Autodesk Inventor part; units mm, degrees
ref_plane "YZ Plane" through (0, 0, 0) normal (1, 0, 0) x (0, 1, 0)
ref_plane "XZ Plane" through (0, 0, 0) normal (0, 1, 0) x (-1, 0, 0)
ref_plane "XY Plane" through (0, 0, 0) normal (0, 0, 1) x (1, 0, 0)
sketch "Sketch1" plane through (0, 0, 0) normal (0, 1, 0) x (-1, 0, 0)
  line L0 (60, -75) -> (-60, -75)
  line L1 (-60, 75) -> (60, -75) construction
  line L2 (60, 75) -> (-60, -75) construction
  line L3 (-60, -75) -> (-60, -55)
  line L4 (-60, -42.5) -> (-60, -55)
  line L5 (0, 75) -> (0, 40)
  line L6 (-60, -75) -> (-60, -5)
  line L7 (-30, 40) -> (-30, 10)
  line L8 (-30, 10) -> (-60, 0)
  line L9 (30, 40) -> (30, 10)
  line L10 (30, 10) -> (60, -5)
  line L11 (-30, 40) -> (-30, 48)
  line L12 (30, 40) -> (30, 48)
  line L13 (0, 75) -> (0, -75)
  line L14 (0, -75) -> (-60, -75)
  line L15 (60, -70) -> (60, -55)
  line L16 (60, -42.5) -> (60, -55)
  line L17 (60, -5) -> (60, -70)
  line L18 (-60, -75) -> (-60, 0)
  line L19 (57, -75) -> (50, -75)
  line L20 (60, -70) -> (60, -75)
  line L21 (-60, -75) -> (-50, -75)
  line L22 (-60, -70) -> (-60, -75)
  line L23 (-60, -70) -> (-50, -75)
  line L24 (60, -70) -> (50, -75)
  line L25 (-27.5, -75) -> (27.5, -75)
  line L26 (27.5, -75) -> (27.5, -5)
  line L27 (27.5, -5) -> (-27.5, -5)
  line L28 (-27.5, -5) -> (-27.5, -75)
  line L29 (30, 10) -> (-30, 10)
  line L30 (0, 75) -> (0, 40)
  line L31 (0, 40) -> (20, 40)
  line L32 (20, 40) -> (-20, 40)
  circle A0 centre (20, 40) radius 1.4
  circle A1 centre (-20, 40) radius 1.4
  line L33 (30, 48) -> (-30, 48)
  line L34 (-60, -75) -> (-35, -75)
  line L35 (60, -75) -> (35, -75)
  line L36 (35, -75) -> (31, -75)
  line L37 (31, -75) -> (31, -67)
  line L38 (31, -67) -> (35, -67)
  line L39 (35, -67) -> (35, -75)
  line L40 (-35, -75) -> (-39, -75)
  line L41 (-39, -75) -> (-39, -67)
  line L42 (-39, -67) -> (-35, -67)
  line L43 (-35, -67) -> (-35, -75)
  circle A2 centre (-35, -67) radius 1.4
  circle A3 centre (31, -67) radius 1.4
  line L44 (30, 48) -> (30, 23)
  line L45 (30, 23) -> (60, -5)
  line L46 (-30, 48) -> (-30, 23)
  line L47 (-30, 23) -> (-60, 0)
  line L48 (-35, -75) -> (-31, -75)
  line L49 (-31, -75) -> (-31, -67)
  line L50 (-31, -67) -> (-35, -67)
  line L51 (-35, -67) -> (-35, -75)
  circle A4 centre (-31, -67) radius 1.4
  dimension "d0" = 120
  dimension "d1" = 150
  dimension "d18" = 70
  dimension "d43" = 55
  dimension "d44" = 70
  dimension "d45" = 35
  dimension "d46" = 20
  dimension "d47" = 40
  dimension "d48" = 2.8
  dimension "d49" = 2.8
  dimension "d50" = 25
  dimension "d51" = 25
  dimension "d52" = 4
  dimension "d53" = 8
  dimension "d54" = 4
  dimension "d55" = 8
  dimension "d56" = 2.8
  dimension "d57" = 2.8
  dimension "d73" = 25
  dimension "d74" = 25
  dimension "d86" = 4
  dimension "d87" = 2.8
extrude "Extrusion1" add sketch "Sketch1" along normal blind 5 contours L24 L0 L39 L38 A3 L37 L26 L27 L13 L29 L10 L17 L16 L15 | L0 L37 A3 L38 L39 | L10 L9 L45 | L0 L13 L27 L26 | L29 L13 L5 L33 L12 L9 | L0 L28 L27 L13 | L29 L7 L11 L33 L5 L13 | L13 L27 L28 L0 L49 A4 L50 A2 L42 L41 L23 L3 L4 L6 L18 L8 L29 | L8 L47 L7 | L0 L43 A2 L50 A4 L49 | L0 L41 L42 A2 L43 | A2 L42 L43 | L43 L50 A2 | L42 A2 L50
fillet "Fillet1" radius 3 8 edges at (30, 2.5, 48) (60, 2.5, 0) (50, 2.5, -75) (60, 2.5, -70) (-60, 2.5, -70) (-50, 2.5, -75) (-60, 2.5, -5) (-30, 2.5, 48)
sketch "Sketch2" plane through (0, 5, 0) normal (0, 1, 0) x (1, 0, 0)
  line L0 (49.2918, 75) -> (-49.2918, 75) construction
  line L1 (0, 75) -> (0, 65) construction
  line L2 (0, 65) -> (30, 65) construction
  circle A0 centre (30, 65) radius 3
  line L3 (0, 75) -> (0, 70)
  line L4 (0, 75) -> (5, 75) construction
  line L5 (0, 58) -> (0, 70)
  line L6 (0, 70) -> (-15, 70)
  line L7 (-15, 70) -> (-15, 61)
  line L8 (-15, 61) -> (0, 61)
  line L9 (0, 61) -> (0, 70)
  line L10 (0, 61) -> (0, -4)
  line L11 (0, -4) -> (-23, -4)
  line L12 (-23, -4) -> (23, -4)
  line L13 (-23, -4) -> (-26, -4)
  line L14 (-26, -4) -> (-26, -24)
  line L15 (-26, -24) -> (-23, -24)
  line L16 (-23, -24) -> (-23, -4)
  line L17 (23, -4) -> (26, -4)
  line L18 (26, -4) -> (26, -24)
  line L19 (26, -24) -> (23, -24)
  line L20 (23, -24) -> (23, -4)
  line L21 (-26, -24) -> (-23, -24)
  line L22 (-23, -24) -> (-23, -14)
  line L23 (-23, -14) -> (-26, -14)
  line L24 (-26, -14) -> (-26, -24)
  line L25 (26, -24) -> (23, -24)
  line L26 (23, -24) -> (23, -14)
  line L27 (23, -14) -> (26, -14)
  line L28 (26, -14) -> (26, -24)
  line L29 (23, -4) -> (-23, -4)
  line L30 (-23, -4) -> (-23, 0)
  line L31 (-23, 0) -> (23, 0)
  line L32 (23, 0) -> (23, -4)
  line L33 (15, 0) -> (-15, 0)
  line L34 (-15, 0) -> (-15, -4)
  line L35 (-15, -4) -> (15, -4)
  line L36 (15, -4) -> (15, 0)
  line L37 (15, 0) -> (-15, -4) construction
  line L38 (-15, 0) -> (15, -4) construction
  point P0 (0, 0)
  point P1 (0, -2)
  dimension "d61" = 10
  dimension "d62" = 30
  dimension "d63" = 6
  dimension "d64" = 5
  dimension "d65" = 90
  dimension "d68" = 15
  dimension "d69" = 9
  dimension "d76" = 65
  dimension "d77" = 23
  dimension "d78" = 46
  dimension "d79" = 3
  dimension "d80" = 20
  dimension "d81" = 3
  dimension "d82" = 20
  dimension "d83" = 10
  dimension "d84" = 10
  dimension "d85" = 30
extrude "Extrusion2" cut sketch "Sketch2" against normal through all contours L8 L7 L6 L5 | L31 L36 L12 L10 | L10 L11 L34 L31 | L16 L15 L14 L23 | L27 L18 L19 L20
properties part number "DeTren"
Part model, mm, in its own coordinate system. A direction names the side the tool comes from. Coordinates: 2 decimals unless noted, no trailing zeros. Order: outer loops, then holes, each group sorted by start corner. A loop starts at its lowest first (then second) coordinate and runs counter-clockwise, first axis right, second up. Notation, with made-up numbers: (79, 16.25) -> (132, 16.25) arc R10 cw to (132, 22.25) -> close; hole circle Ø6 at (68, 4). An arc over 180 degrees is marked (long way). Put each result on its own line as item: value. Start each with the question number.
(1) Band-saw the part on A-A (z = 40). Give the cut face in (x, y), then the cut area to 3 significant figures.
(2) Band-saw the part on B-B (x = -20). Give the cut face in (y, z).
(3) Probe line 1 along Z through (x, y) = (-8, 4.6); line 2 along Z through (x, y) = (20, 1.45); line 3 along Z through (x, y) = (1, 3.3). List the from-to ranges inside material, lowest first. Write a range as [from, to].
(4) Band-saw the part on D-D (z = 9). Give the cut face in (x, y), then the cut area to 3 significant figures.
(5) Band-saw the part on C-C (y = 4.05). Count the separate pieces of the cut face and the enclosed holes in it, then the cut area to 3 significant figures.
(6) Mould opens along Z. For faces 1 (the face through (44.211, 2.465, 12.105)), 2 (the face through (-30, 2, 34)), 3 (the face through (24, 3, 14)), 4 (the face through (-54.54, 2.46, -72.73)) say: pulls with the +Z half, pulls with the -Z half, needs draft (parallel to the pull), parting line crosses it, or undercut.
(7) Which spindle directions (+Z, -Z, +X, -X, +Y, -Y) get a long thin tool onto all of the face, cutting with end or side? Do faces 5 (the face through (60, 2, -35)), 6 (the face through (-23, 3, 19)). Say none if no direction does.
(8) Pin check, flat tips, straight feed: pin 1 Ø2.5 at (y, z) = (2.5, 18.5) entering from -X; pin 2 Ø1.7 at (x, z) = (31, -67) entering from -Y; pin 3 Ø2.5 at (y, z) = (3.5, 35.5) entering from -X; pin 4 Ø3 at (y, z) = (2.5, 2.5) entering from +X. Stop position of each tip, or through.
Determined:
1. outline: (-30, 0) -> (-21.4, 0) -> (-21.4, 5) -> (-30, 5) -> close; (-18.6, 0) -> (18.6, 0) -> (18.6, 5) -> (-18.6, 5) -> close; (21.4, 0) -> (30, 0) -> (30, 5) -> (21.4, 5) -> close
1. area: 272 mm²
2. outline: (0, -75) -> (5, -75) -> (5, 38.6) -> (0, 38.6) -> close; (0, 41.4) -> (5, 41.4) -> (5, 48) -> (0, 48) -> close
3. line 1: z = [-75, -70], [-61, 0], [4, 48]
3. line 2: z = [-75, 38.6], [41.4, 48]
3. line 3: z = [-75, 0], [4, 48]
4. outline: (-45, 0) -> (48.26, 0) -> (48.26, 5) -> (-45, 5) -> close
4. area: 466 mm²
5. separate pieces: 1
5. enclosed holes: 8
5. area: 12,100 mm²
6. face 1: pulls with the +Z half
6. face 2: needs draft
6. face 3: undercut
6. face 4: pulls with the -Z half
7. face 5: +Z, -Z, +X, +Y, -Y
7. face 6: +Y, -Y
8. pin 1: stops at x = -36.16
8. pin 2: passes through
8. pin 3: stops at x = -30
8. pin 4: stops at x = 58.7
